The model under review builds one solid part; all positions refer to its coordinate system, in mm. A direction names the side the tool comes from. Round coordinates to 2 decimals unless told otherwise and drop trailing zeros. Order: outer loops, then holes, each group sorted by start corner. A loop starts at its lowest first (then second) coordinate and runs counter-clockwise, first axis right, second up. Notation, with made-up numbers: M 68,28 L 90,28 A28 ccw 90,56 Z; hole C 18,59.25 d6. An arc over 180 degrees is marked long. Answer as a JSON object with one key per item and string values. Group by question number.
1) The part is to be moulded in two halves that separate along Y. For faces 4 (the flat face through (1, 3, -6.7)), 5 (the flat face through (1, 1, -3)), 6 (the cylindrical face through (-4.46, -0.59, -5.46)), say which applies: +Y half, -Y half, draft (parallel to the pull), parting line (faces both ways), or undercut.
2) Consider section B-B, the plane x = 0. Count the separate pieces of the cut face and the enclosed holes in it, then the cut area to 3 significant figures.
3) Consider section A-A, the plane z = -2.25. Write out the cut boundary in (x, y).
4) To check wall thickness, follow line 1 (X direction, y = 0, z = -1.25); line 2 (X direction, y = 0, z = -2.2). State the ranges of each line that lie inside material, in increasing order.
5) Insertion check: pin 1 Ø5 at (x, y) = (0, 0) entering from +Z; pin 2 Ø1.4 at (x, y) = (8, 0) entering from +Z; pin 3 Ø2 at (x, y) = (-8, 0) entering from +Z; pin 4 Ø1 at (y, z) = (-1, -2.5) entering from -X. Each pin has a flat end and moves straight along its axis. Give the tip position at first contact, or say it passes through.
6) For faces 1 (the flat face through (1, -1, -1.5)), 2 (the flat face through (5, 0, -4.5)), 3 (the cylindrical face through (1.22, -0.27, -2.24)), list the 3-axis set-ups (+Z, -Z, +X, -X, +Y, -Y) from which the entire face can be reached by the end or side of a thin tool; tool diameter is ignored.
7) Consider section C-C, the plane z = -5.25. Write out the cut boundary in (x, y).
```python
from build123d import *

# Parameters (mm, degrees)
M2_TAPPED_HOLE1_AT_2_COUNT = 2
M2_TAPPED_HOLE1_AT_2_PITCH = 11.313708499
M2_TAPPED_HOLE1_AT_3_COUNT = 2
M2_TAPPED_HOLE1_AT_3_PITCH = 16
M2_TAPPED_HOLE1_AT_4_COUNT = 2
M2_TAPPED_HOLE1_AT_4_PITCH = 11.313708499
M2_TAPPED_HOLE1_AT_5_COUNT = 2
M2_TAPPED_HOLE1_AT_5_PITCH = 8
CHAMFER1_SIZE              = 0.3


with BuildPart() as part:
    # Sketch1 → Revolve1 (revolve)
    with BuildSketch(Plane(origin=(0, 0, 0), x_dir=(0, 0, -1), z_dir=(1, 0, 0))):
        Polygon((3, 1.25), (1.5, 1.25), (1.5, 2.75), (0, 2.75), (0, 11), (4.5, 11), (4.5, 4.5), (6.7, 4.5), (6.7, 2.75), (3, 2.75), align=None)
    revolve(axis=Axis((0, 0, 0), (0, 0, 1)))

    # Sketch4 → M2 Tapped Hole1 (revolve, cut)
    with BuildSketch(Plane(origin=(0, 8, 0), x_dir=(0, -1, 0), z_dir=(1, 0, 0))):
        Polygon((0, 0), (0, 4.5), (1.025, 4.5), (0.8, 4.370096189), (0.8, 0.129903811), (1.025, 0), align=None)
    m2_tapped_hole1 = revolve(axis=Axis((0, 8, 6.35), (0, 0, -1)), mode=Mode.SUBTRACT)

    # M2 Tapped Hole1 at 2: M2 Tapped Hole1 ×2
    with Locations(*[Vector(0.707106781, -0.707106781, 0) * (i * M2_TAPPED_HOLE1_AT_2_PITCH) for i in range(1, M2_TAPPED_HOLE1_AT_2_COUNT)]):
        add(m2_tapped_hole1, mode=Mode.SUBTRACT)

    # M2 Tapped Hole1 at 3: M2 Tapped Hole1 ×2
    with Locations(*[(0, -i * M2_TAPPED_HOLE1_AT_3_PITCH, 0) for i in range(1, M2_TAPPED_HOLE1_AT_3_COUNT)]):
        add(m2_tapped_hole1, mode=Mode.SUBTRACT)

    # M2 Tapped Hole1 at 4: M2 Tapped Hole1 ×2
    with Locations(*[Vector(-0.707106781, -0.707106781, 0) * (i * M2_TAPPED_HOLE1_AT_4_PITCH) for i in range(1, M2_TAPPED_HOLE1_AT_4_COUNT)]):
        add(m2_tapped_hole1, mode=Mode.SUBTRACT)

    # M2 Tapped Hole1 at 5: M2 Tapped Hole1 ×2
    with Locations(*[(0, -i * M2_TAPPED_HOLE1_AT_5_PITCH, 0) for i in range(1, M2_TAPPED_HOLE1_AT_5_COUNT)]):
        add(m2_tapped_hole1, mode=Mode.SUBTRACT)

    # Chamfer1
    chamfer1_edges = [part.edges().sort_by_distance(p)[0] for p in [
        (0, -11, -4.5),
        (0, -11, 0),
        (0, -2.75, 0),
        (0, -4.5, -6.7),
    ]]
    chamfer(chamfer1_edges, length=CHAMFER1_SIZE)


solid = part.part
```
Results list:
{
 "1": {"face 4": "draft", "face 5": "undercut", "face 6": "parting line"},
 "2": {"separate pieces": "4", "enclosed holes": "0", "area": "71.6 mm^2"},
 "3": {"outline": "C 0,0 d22; hole C -8,0 d1.6; hole C 0,0 d2.5; hole C 0,-8 d1.6; hole C 0,8 d1.6; hole C 8,0 d1.6"},
 "4": {"line 1": "-11 to -8.8, -7.2 to -2.75, 2.75 to 7.2, 8.8 to 11", "line 2": "-11 to -8.8, -7.2 to -1.25, 1.25 to 7.2, 8.8 to 11"},
 "5": {"pin 1": "z = -1.5", "pin 2": "through", "pin 3": "z = -0.01", "pin 4": "x = -10.99"},
 "6": {"face 1": "+Z", "face 2": "-Z", "face 3": "+Z, -Z"},
 "7": {"outline": "C 0,0 d9; hole C 0,0 d5.5"}
}
